Input: part model. Units: mm. Frame: model coordinates. A direction names the side the tool comes from. Round coordinates to 2 decimals unless told otherwise and drop trailing zeros. Order: outer loops, then holes, each group sorted by start corner. A loop starts at its lowest first (then second) coordinate and runs counter-clockwise, first axis right, second up.
Item 1: Cut plane B-B on y = 59. Output: boundary loops of the cut face in (x, z) (3 decimals), then the cut area to 3 significant figures.
Item 2: First-contact query: pin 1 (1 mm diameter, centred on x = -53.5, y = 2, fed in from -Z) (3 decimals); pin 2 (4 mm diameter, centred on x = -8, y = 106.5, fed in from +Z); pin 3 (6.5 mm diameter, centred on x = 9, z = 19, fed in from +Y) (3 decimals). Flat tips, straight axial feed; report the tip coordinate or a pass-through.
Item 3: Mould query, pull axis X, two halves, no side actions, for faces 1 (the cylindrical face through (53.82, 1.57, 16.61)), 2 (the cylindrical face through (-61.689, 1.565, 5.085)), 3 (the flat face through (-1, 3.175, 14)), 4 (the cylindrical face through (61.59, 1.57, 23.59)). Classes: released by +X, released by -X, zero draft, split by the parting line, or undercut.
Item 4: Line query: L1, parallel to Y at x = 58.5, z = 23.5 (3 decimals); L2, parallel to Z at x = 5, y = 107 (3 decimals); L3, parallel to Y at x = 21, z = -1.5. Output: solid intervals per line, ascending.
Item 5: Cut plane A-A on x = -29. Output: boundary loops of the cut face in (y, z) (3 decimals).
Item 6: Reachability of faces 5 (the flat face through (-1, 129, 0)), 6 (the flat face through (-1, 0, 14)) from +Z, -Z, +X, -X, +Y, -Y: full face, straight path, thin tool, end or side. Return the list, or none.
```python
from build123d import *

# Parameters (mm, degrees)
SKETCH1_W                    = 101.6
SKETCH1_H                    = 247.65
BASE_FLANGE1_DEPTH           = 3.175
EDGE_FLANGE1_STRIP_W         = 19.05
EDGE_FLANGE1_STRIP_H         = 3.175
EDGE_FLANGE1_STRIP_CUT_DEPTH = 101.6
EDGE_FLANGE1_DEPTH           = 101.6
FILLET1_R                    = 12.7
SKETCH9_W                    = 127
SKETCH9_H                    = 22.225
BOSS_EXTRUDE1_DEPTH          = 3.175
F_1_4_CLEARANCE_HOLE1_D      = 7.62
FILLET3_R                    = 6.35


# Sheet-metal steps are written as plain solids
with BuildPart() as part:
    # Sketch1 → Base-Flange1 (new body)
    with BuildSketch(Plane.XY):
        with Locations((0, 123.825)):
            Rectangle(SKETCH1_W, SKETCH1_H)
    extrude(amount=-BASE_FLANGE1_DEPTH)

    # Edge-Flange1 strip (across the edge) → Edge-Flange1 strip cut (cut)
    with BuildSketch(Plane.YZ.offset(-50.8)):
        with Locations((-3.175, -1.5875)):
            Rectangle(EDGE_FLANGE1_STRIP_W, EDGE_FLANGE1_STRIP_H)
    extrude(amount=EDGE_FLANGE1_STRIP_CUT_DEPTH, mode=Mode.SUBTRACT)

    # Edge-Flange1 section (across the edge) → Edge-Flange1 (add)
    with BuildSketch(Plane.YZ.offset(-50.8)):
        with BuildLine():
            Line((0, 3.175), (0, 25.4))
            Line((0, 25.4), (3.175, 25.4))
            Line((3.175, 25.4), (3.175, 3.175))
            ThreePointArc((3.175, 3.175), (4.10493597, 0.92993597), (6.35, 0))
            Line((6.35, 0), (6.35, -3.175))
            ThreePointArc((6.35, -3.175), (1.859871939, -1.315128061), (0, 3.175))
        make_face()
    extrude(amount=EDGE_FLANGE1_DEPTH)

    # Fillet1
    fillet1_edges = [part.edges().sort_by_distance(p)[0] for p in [
        (-50.8, 247.65, -1.5875),
        (50.8, 247.65, -1.5875),
    ]]
    fillet(fillet1_edges, radius=FILLET1_R)

    # Sketch9 → Boss-Extrude1 (add)
    with BuildSketch(Plane(origin=(0, 3.175, 0), x_dir=(1, 0, 0), z_dir=(0, 1, 0))):
        with Locations((0, -14.2875)):
            Rectangle(SKETCH9_W, SKETCH9_H)
    extrude(amount=-BOSS_EXTRUDE1_DEPTH)

    # 1/4 Clearance Hole1 (through all)
    with Locations(Plane(origin=(0, 3.175, 0), x_dir=(1, 0, 0), z_dir=(0, 1, 0))):
        with Locations((-50.8, -14.2875), (50.8, -14.2875)):
            Hole(F_1_4_CLEARANCE_HOLE1_D / 2)

    # Fillet3
    fillet3_edges = [part.edges().sort_by_distance(p)[0] for p in [
        (-63.5, 1.5875, 3.175),
        (63.5, 1.5875, 25.4),
        (-63.5, 1.5875, 25.4),
        (63.5, 1.5875, 3.175),
    ]]
    fillet(fillet3_edges, radius=FILLET3_R)


solid = part.part
```
From the geometry:
1. outline: (-50.8, -3.175) - (50.8, -3.175) - (50.8, 0) - (-50.8, 0) - close
1. area: 323 mm2
2. pin 1: stops at z = 3.175
2. pin 2: stops at z = 0
2. pin 3: stops at y = 3.175
3. face 1: undercut
3. face 2: released by -X
3. face 3: zero draft
3. face 4: released by +X
4. L1: y = 0 to 3.175
4. L2: z = -3.175 to 0
4. L3: y = 2.05 to 247.65
5. outline: (0, 3.175) arc R6.35 ccw to (6.35, -3.175) - (247.65, -3.175) - (247.65, 0) - (6.35, 0) arc R3.175 cw to (3.175, 3.175) - (3.175, 25.4) - (0, 25.4) - close
6. face 5: +Z, +X, -X, +Y
6. face 6: +Z, -Z, +X, -X, -Y
